For this review, take the finished solid that the model builds, in its own axes (mm). A direction names the side the tool comes from. Give positions to 0.01 mm unless a question says otherwise; leave off trailing zeros. Loops run counter-clockwise (first coordinate to the right, second up) from the corner with the lowest first, then second, coordinate; pieces in that order, holes last. Notation, with made-up numbers: (80.5, 80) - (99.5, 80) arc R12 ccw to (99.5, 98) - close; hole circle Ø6 at (60.5, -12.75). An arc over 180 degrees is marked (long way). Answer in a Markdown table with one row per item.
```python
from build123d import *

# Parameters (mm, degrees)
SKETCH1_R           = 9.525
BOSS_EXTRUDE1_DEPTH = 25.4
SKETCH3_R           = 30.353
BOSS_EXTRUDE2_DEPTH = 397.764
SKETCH4_R           = 32.893
BOSS_EXTRUDE3_DEPTH = 2.54


with BuildPart() as part:
    # Sketch1 → Boss-Extrude1 (new, symmetric)
    with BuildSketch(Plane.XY):
        with BuildLine():
            Line((-123.19, -150.1775), (-123.19, 150.1775))
            ThreePointArc((-123.19, 150.1775), (-108.311024484, 186.098524484), (-72.39, 200.9775))
            Line((-72.39, 200.9775), (27.6225, 200.9775))
            Line((27.6225, 200.9775), (27.6225, 251.7775))
            Line((27.6225, 251.7775), (-11.443122974, 284.057790065))
            ThreePointArc((-11.443122974, 284.057790065), (-30.027308672, 289.763403093), (-47.202790065, 280.656877026))
            Line((-47.202790065, 280.656877026), (-71.066089722, 251.7775))
            Line((-71.066089722, 251.7775), (-72.39, 251.7775))
            ThreePointArc((-72.39, 251.7775), (-144.232048969, 222.019548969), (-173.99, 150.1775))
            Line((-173.99, 150.1775), (-173.99, -150.1775))
            Line((-173.99, -150.1775), (-123.19, -150.1775))
        make_face()
        with Locations((-27.6225, 264.4775)):
            Circle(SKETCH1_R, mode=Mode.SUBTRACT)
    extrude(amount=BOSS_EXTRUDE1_DEPTH, both=True)

    # Sketch2 → Revolve1 (revolve)
    with BuildSketch(Plane.XZ.offset(150.1775)):
        Polygon((-173.99, 0), (-123.19, 0), (-55.245, 0), (-55.245, 129.159), (-80.645, 129.159), (-80.645, 25.4), (-123.19, 25.4), (-123.19, 40.719375), (-173.99, 40.719375), align=None)
    revolve(axis=Axis((-173.99, -150.1775, 0), (1, 0, 0)))

    # Sketch3 → Boss-Extrude2 (add)
    with BuildSketch(Plane.XZ.offset(-200.9775)):
        with Locations(Location((27.6225, 0, 0), (0, 0, 236.805836124))):
            Circle(SKETCH3_R)
    extrude(amount=-BOSS_EXTRUDE2_DEPTH)

    # Sketch4 → Boss-Extrude3 (add)
    with BuildSketch(Plane(origin=(0, 340.6775, 0), x_dir=(1, 0, 0), z_dir=(0, 1, 0))):
        with Locations(Location((27.6225, 0, 0), (0, 0, 270))):
            Circle(SKETCH4_R)
    extrude(amount=-BOSS_EXTRUDE3_DEPTH)


solid = part.part
```
1. Mouldability with a two-part tool opening along Y and no side actions: class faces 1 (the face through (-2.58, 467.9, 3.02)), 2 (the face through (57.037, 268.597, 7.49)), 3 (the face through (28, 598.742, 0)) as released by +Y, released by -Y, zero draft, split by the parting line, or undercut.
Values:
| item | result |
|---|---|
| face 1 | zero draft |
| face 2 | undercut |
| face 3 | released by +Y |
2. Wall thickness on line 1 (Y direction, x = 48.5, z = 14.5); line 2 (X direction, y = -47.5, z = 57.5) (3 decimals); line 3 (X direction, y = -144.5, z = -21) (3 decimals): over which ranges is each line inside the solid? List them lowest first. Write a range as [from, to].
Values:
| item | result |
|---|---|
| line 1 | y = [200.98, 598.74] |
| line 2 | x = [-80.645, -55.245] |
| line 3 | x = [-173.99, -55.245] |
3. We need section A-A, the plane y = -106.5. Give the boundary of the cut face in (x, z) (3 decimals), and give its area (3 significant figures).
Values:
| item | result |
|---|---|
| outline | (-173.99, -25.4) - (-123.19, -25.4) - (-123.19, 25.4) - (-173.99, 25.4) - close; (-80.645, -121.55) - (-55.245, -121.55) - (-55.245, 121.55) - (-80.645, 121.55) - close |
| area | 8,760 mm^2 |
4. We need section D-D, the plane y = 34. Give the boundary of the cut face in (x, z), and give its area (3 significant figures).
Values:
| item | result |
|---|---|
| outline | (-173.99, -25.4) - (-123.19, -25.4) - (-123.19, 25.4) - (-173.99, 25.4) - close |
| area | 2,580 mm^2 |
5. For faces 4 (the face through (-108.704, 185.701, 0.356)), 5 (the face through (18, 340.678, 29)), 6 (the face through (18, 338.138, 29)), 7 (the face through (-173.99, -23, -1)), 8 (the face through (-55.245, -152, 2)), list the 3-axis set-ups (+Z, -Z, +X, -X, +Y, -Y) from which the entire face can be reached by the end or side of a thin tool; tool diameter is ignored.
Values:
| item | result |
|---|---|
| face 4 | +Z, -Z, +X |
| face 5 | +Y |
| face 6 | none |
| face 7 | +Z, -Z, -X, +Y, -Y |
| face 8 | +Z, -Z, +X, -Y |
6. Clearance check with flat-ended pins moving along their axes: pin 1 (3 mm diameter, centred on x = -31, z = 15, fed in from +Y); pin 2 (8 mm diameter, centred on y = 27, z = -26.5, fed in from +X); pin 3 (25 mm diameter, centred on x = -27.62, y = 264.48, fed in from -Z). State where each tip first meets the part, or that it passes through.
Values:
| item | result |
|---|---|
| pin 1 | stops at y = 289.81 |
| pin 2 | stops at x = -123.19 |
| pin 3 | stops at z = -25.4 |
7. We need section C-C, the plane x = 45. Give the boundary of the cut face in (y, z).
Values:
| item | result |
|---|---|
| outline | (200.98, -24.89) - (338.14, -24.89) - (338.14, -27.93) - (340.68, -27.93) - (340.68, -24.89) - (598.74, -24.89) - (598.74, 24.89) - (340.68, 24.89) - (340.68, 27.93) - (338.14, 27.93) - (338.14, 24.89) - (200.98, 24.89) - close |
